from build123d import *

# Parameters (mm, degrees)
SKETCH_2_R          = 2.5
EXTRUDE_1_DEPTH     = 6
SKETCH_3_R          = 1.6
CUT_EXTRUDE_1_DEPTH = 10
SKETCH_4_R          = 1.6
CUT_EXTRUDE_2_DEPTH = 20


with BuildPart() as part:
    # 草图2 → 凸台-拉伸1 (new body)
    with BuildSketch(Plane.XY):
        with BuildLine():
            Line((-37.476659403, -37.476659403), (-35.355339059, -35.355339059))
            Line((-35.355339059, -35.355339059), (-34.635011938, -18.618967428))
            Line((-34.635011938, -18.618967428), (-30.804789722, -15.40502938))
            Line((-30.804789722, -15.40502938), (-28.233639283, -18.469207152))
            Line((-28.233639283, -18.469207152), (-22.871328181, -13.969693884))
            Line((-22.871328181, -13.969693884), (-25.44247862, -10.905516112))
            Line((-25.44247862, -10.905516112), (-26.72805384, -9.373427226))
            Line((-26.72805384, -9.373427226), (-37.149566653, -2.1420772))
            ThreePointArc((-37.149566653, -2.1420772), (-41.092578269, -1.370832784), (-44.330127019, -3.75))
            Line((-44.330127019, -3.75), (-50.830440783, -15.008873704))
            ThreePointArc((-50.830440783, -15.008873704), (-45.560249498, -27.07884166), (-37.476659403, -37.476659403))
        make_face()
        with Locations((-40, -6.25)):
            Circle(SKETCH_2_R, mode=Mode.SUBTRACT)
    extrude(amount=EXTRUDE_1_DEPTH)

    # 草图3 → 切除-拉伸1 (cut)
    with BuildSketch(Plane(origin=(0, 0, 0), x_dir=(-1, 0, 0), z_dir=(0, 0, -1))):
        with Locations((42.582783582, -23.873668727)):
            Circle(SKETCH_3_R)
        with Locations((38, -32)):
            Circle(SKETCH_3_R)
    extrude(amount=-CUT_EXTRUDE_1_DEPTH, mode=Mode.SUBTRACT)

    # 草图4 → 切除-拉伸2 (cut)
    with BuildSketch(Plane(origin=(-2.571150439, 3.064177772, 0), x_dir=(0.7660444431189767, 0.642787609686541, 0), z_dir=(0.642787609686541, -0.7660444431189767, 0))):
        with Locations((-30, 3)):
            Circle(SKETCH_4_R)
    extrude(amount=-CUT_EXTRUDE_2_DEPTH, mode=Mode.SUBTRACT)


solid = part.part
Source: CAD feature listing. Evaluate the final solid. Frame: model axes, mm. A direction names the side the tool comes from. Give positions to 0.01 mm unless a question says otherwise; leave off trailing zeros. Write each loop counter-clockwise with the first axis right and the second up, starting at its lowest first coordinate (ties: lowest second). Pieces come first, ordered by that corner, then holes. Notation, with made-up numbers: M 31,68 L 89,68 A30 ccw 89,90 Z; hole C 45,21.5 d4. An arc over 180 degrees is marked long. Return JSON: item names as keys, results as strings. Group by question number.
1) Set-up query: faces 4 (the face through (-37.69, -7.21, 2.96)), 5 (the face through (-29.537, -16.916, 2.958)). Return all of +Z, -Z, +X, -X, +Y, -Y with unobstructed straight access to the full face (end or side cutting, diameter ignored); none if empty.
2) Cut plane A-A, the plane y = -32. Output: boundary loops of the cut face in (x, z).
3) Draft query along X for faces 1 (the face through (-36, -36, 3)), 2 (the face through (-32.747, -17.034, 2.958)), 3 (the face through (-37, -15, 6)). Return one class per face: released by +X, released by -X, zero draft, split by the parting line, or undercut.
4) Ray query, L1, parallel to X at y = -6.5, z = 1.75; L2, parallel to Y at x = -38, z = 2.25; L3, parallel to X at y = -4, z = 1. Return the intervals inside material, ascending.
5) First-contact query: pin 1 Ø1 at (x, z) = (-45.5, 2.5) entering from -Y; pin 2 Ø3 at (y, z) = (-26.5, 1) entering from -X; pin 3 Ø1 at (x, z) = (-43, 0.5) entering from +Y. Flat tips, straight axial feed; report the tip coordinate or a pass-through.
6) Cut plane B-B, the plane x = -38. Give the number of separate pieces and of enclosed holes in the cut face, then the cut area to 3 significant figures.
7) Cut plane D-D, the plane x = -48.5. Output: boundary loops of the cut face in (y, z).
Data:
{
 "1": {"face 4": "+Z, -Z", "face 5": "+Z, -Z, -Y"},
 "2": {"outline": "M -42.25,0 L -39.6,0 L -39.6,6 L -42.25,6 Z; M -36.4,0 L -35.21,0 L -35.21,6 L -36.4,6 Z"},
 "3": {"face 1": "released by +X", "face 2": "undercut", "face 3": "zero draft"},
 "4": {"L1": "x = -45.92 to -42.49, -37.51 to -35.01, -32.4 to -30.87", "L2": "y = -36.95 to -33.6, -30.4 to -7.75, -4.75 to -3.58", "L3": "x = -44.47 to -41.09, -38.91 to -34.47"},
 "5": {"pin 1": "stops at y = -28", "pin 2": "stops at x = -46.73", "pin 3": "stops at y = -1.92"},
 "6": {"separate pieces": "3", "enclosed holes": "0", "area": "169 mm²"},
 "7": {"outline": "M -21.37,0 L -10.97,0 L -10.97,6 L -21.37,6 Z"}
}
